For this review, use the dimensioned drawing (mm, ordinates from the lowest corner) and the shaded views. A direction names the side the tool comes from. Give positions to 0.01 mm unless a question says otherwise; leave off trailing zeros. Write each loop counter-clockwise with the first axis right and the second up, starting at its lowest first coordinate (ties: lowest second). Pieces come first, ordered by that corner, then holes.
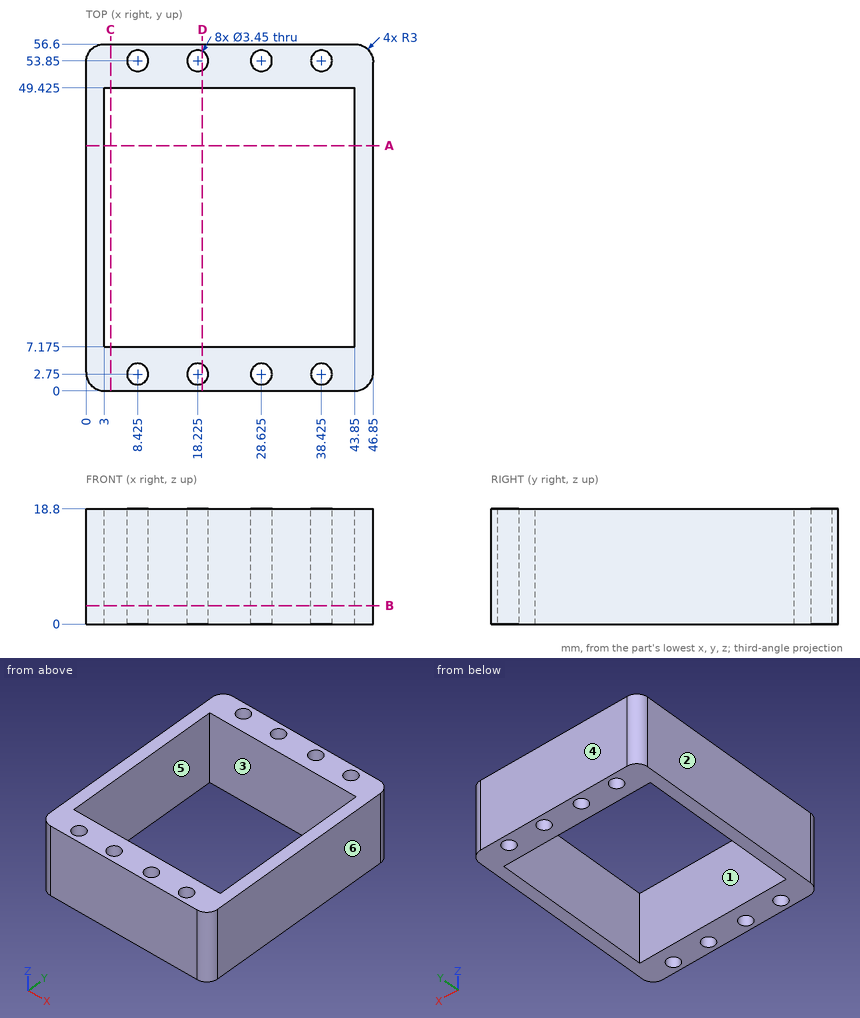
(1) We need section B-B (z = 3). Count the separate pieces of the cut face and the enclosed holes in it, and give its area (3 significant figures).
(2) We need section D-D (x = 19). Write out the cut boundary in (y, z) (3 decimals).
(3) We need section C-C (x = 4). Write out the cut boundary in (y, z) (3 decimals).
(4) For L1, parallel to X at y = 53.85, z = 11; L2, parallel to X at y = 46.5, z = 3.5; L3, parallel to Y at x = 28.5, z = 5.75 (3 decimals), list the stretches that pass through material, from the lowest coordinate up.
(5) The part is to be moulded in two halves that separate along Y. For the marked faces 3, 4, 5 and 6, say which applies: +Y half, -Y half, draft (parallel to the pull), parting line (faces both ways), or undercut.
(6) Tool access review of the marked faces 1 and 2: name each direction out of +Z, -Z, +X, -X, +Y, -Y from which nothing blocks a thin tool from reaching the whole face with its end or side.
(7) We need section A-A (y = 40). Write out the cut boundary in (x, z), and give its area (3 significant figures).
(8) Clearance check with a flat-ended pin moving along its axis: pin 1 Ø2 at (x, y) = (28.625, 2.75) entering from +Z. State where the tip first meets the part, or that it passes through.
The answers:
1. separate pieces: 1
1. enclosed holes: 9
1. area: 843 mm2
2. outline: (0, 0) - (1.209, 0) - (1.209, 18.8) - (0, 18.8) - close; (4.291, 0) - (7.175, 0) - (7.175, 18.8) - (4.291, 18.8) - close; (49.425, 0) - (52.309, 0) - (52.309, 18.8) - (49.425, 18.8) - close; (55.391, 0) - (56.6, 0) - (56.6, 18.8) - (55.391, 18.8) - close
3. outline: (0, 0) - (7.175, 0) - (7.175, 18.8) - (0, 18.8) - close; (49.425, 0) - (56.6, 0) - (56.6, 18.8) - (49.425, 18.8) - close
4. L1: x = 0.01 to 6.7, 10.15 to 16.5, 19.95 to 26.9, 30.35 to 36.7, 40.15 to 46.84
4. L2: x = 0 to 3, 43.85 to 46.85
4. L3: y = 0 to 1.03, 4.47 to 7.175, 49.425 to 52.13, 55.57 to 56.6
5. face 3: undercut
5. face 4: +Y half
5. face 5: undercut
5. face 6: draft
6. face 1: +Z, -Z
6. face 2: +Z, -Z, -X, +Y, -Y
7. outline: (0, 0) - (3, 0) - (3, 18.8) - (0, 18.8) - close; (43.85, 0) - (46.85, 0) - (46.85, 18.8) - (43.85, 18.8) - close
7. area: 113 mm2
8. pin 1: passes through
